```python
from build123d import *

# Parameters (mm, degrees)
F0_W     = 40
F0_H     = 40
F1_DEPTH = 30
F3_DEPTH = 20
F2_W     = 40
F2_H     = 6.755145
F4_DEPTH = 30.001


with BuildPart() as f1:
    # F0 (on Top) → F1 (new body)
    with BuildSketch(Plane.XY):
        Rectangle(F0_W, F0_H)
    extrude(amount=-F1_DEPTH)

    # F2 (on face) → F3 (cut)
    with BuildSketch(Plane.XY):
        Polygon((20, -10.641778), (20, 0), (0, 7.279405), (-20, 0), (-20, -10.641778), (0, -3.362373), align=None)
    extrude(amount=-F3_DEPTH, mode=Mode.SUBTRACT)

    # F2 (on face) → F4 (cut, through all)
    with BuildSketch(Plane.XY):
        Polygon((-20, -20), (20, -20), (0, -12.720595), align=None)
        with Locations((0, 16.622428)):
            Rectangle(F2_W, F2_H)
    extrude(amount=-F4_DEPTH, mode=Mode.SUBTRACT)


solid = f1.part
```
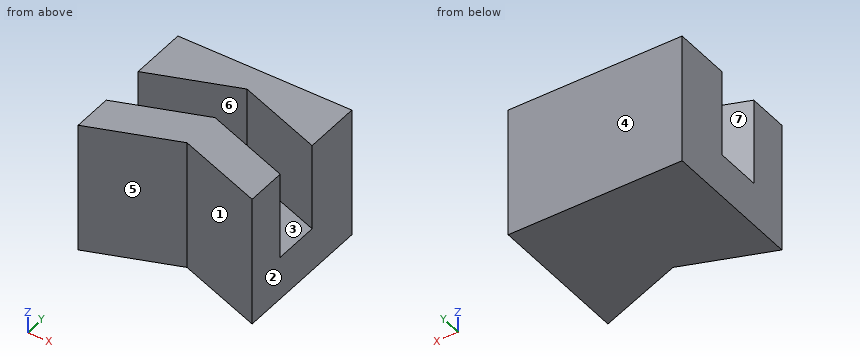
Read the model definition and answer for the solid it produces. Units are mm, in the model's axes. Face numbers are marked on the shaded views. A direction names the side the tool comes from. Coordinates: 2 decimals unless noted, no trailing zeros. Write each loop counter-clockwise with the first axis right and the second up, starting at its lowest first coordinate (ties: lowest second). Pieces come first, ordered by that corner, then holes. Notation, with made-up numbers: (-24, 49) -> (-5, 49) arc R11 ccw to (-5, 59) -> close; hole circle Ø4 at (37.25, 20). An arc over 180 degrees is marked (long way). Answer as a JSON object with one key per item and string values.
Q1. Determine the mould class of the marked faces 1, 2, 3 and 4 for opening direction Y: pulls with the +Y half, pulls with the -Y half, needs draft (parallel to the pull), parting line crosses it, or undercut.
The answers:
{"face 1": "pulls with the -Y half", "face 2": "needs draft", "face 3": "undercut", "face 4": "pulls with the +Y half"}
Q2. The part is cut by section B-B on y = -15. Give the vertices of the cut face in (x, z).
The answers:
{"outline": "(-20, -30) -> (-6.26, -30) -> (-6.26, 0) -> (-20, 0) -> close; (6.26, -30) -> (20, -30) -> (20, 0) -> (6.26, 0) -> close"}
Q3. The part is cut by section D-D on z = -25.5. Give the vertices of the cut face in (x, y).
The answers:
{"outline": "(-20, -20) -> (0, -12.72) -> (20, -20) -> (20, 13.24) -> (-20, 13.24) -> close"}
Q4. The part is cut by section C-C on x = -17. Give the vertices of the cut face in (y, z).
The answers:
{"outline": "(-18.91, -30) -> (13.24, -30) -> (13.24, 0) -> (1.09, 0) -> (1.09, -20) -> (-9.55, -20) -> (-9.55, 0) -> (-18.91, 0) -> close"}
Q5. A tool of negligible diameter and unlimited length cuts with its end or side. For the marked faces 5, 6 and 7, from which of +Z, -Z, +X, -X, +Y, -Y can it reach the whole face along a straight path? Write none if from no direction.
The answers:
{"face 5": "+Z, -Z, -Y", "face 6": "+Z", "face 7": "+Z, -X"}
Q6. Consider line 1 (Y direction, x = -12, z = -2); line 2 (Y direction, x = -5, z = -1.5); line 3 (Z direction, x = 14.5, y = -6). Determine where each line is inside the solid, lowest interval first. Write a range as [from, to].
The answers:
{"line 1": "y = [-17.09, -7.73], [2.91, 13.24]", "line 2": "y = [-14.54, -5.18], [5.46, 13.24]", "line 3": "z = [-30, -20]"}
Q7. Flat-ended cylindrical pins translate along their axes: pin 1 Ø6 at (x, z) = (-5, -5) entering from -Y; pin 2 Ø1 at (x, z) = (-1.5, -23) entering from -Y; pin 3 Ø1.5 at (x, z) = (-4, -13.5) entering from -Y. Find the tip coordinate at first contact, or state that the pin passes through.
The answers:
{"pin 1": "stops at y = -15.63", "pin 2": "stops at y = -13.45", "pin 3": "stops at y = -14.45"}
Q8. The part is cut by section A-A on z = -18.5. Give the vertices of the cut face in (x, y).
The answers:
{"outline": "(-20, -20) -> (0, -12.72) -> (20, -20) -> (20, -10.64) -> (0, -3.36) -> (-20, -10.64) -> close; (-20, 0) -> (0, 7.28) -> (20, 0) -> (20, 13.24) -> (-20, 13.24) -> close"}
